The model under review builds one solid part; all positions refer to its coordinate system, in mm. A direction names the side the tool comes from. Coordinates: 2 decimals unless noted, no trailing zeros. Order: outer loops, then holes, each group sorted by start corner. A loop starts at its lowest first (then second) coordinate and runs counter-clockwise, first axis right, second up. Notation, with made-up numbers: (-36, -36) -> (18, -36) arc R23 cw to (18, -17) -> close; hole circle Ø3 at (40.5, 19.25). An arc over 180 degrees is marked (long way). Put each result on its own line as item: value.
from build123d import *

# Parameters (mm, degrees)
SKETCH1_R           = 11.875
SKETCH1_R_2         = 5
BOSS_EXTRUDE1_DEPTH = 11
CUT_EXTRUDE1_DEPTH  = 21.075638221
SKETCH4_R           = 13.875
SKETCH4_R_2         = 5
BOSS_EXTRUDE2_DEPTH = 1
LPATTERN1_COUNT     = 2
LPATTERN1_PITCH     = 12


with BuildPart() as part:
    # Sketch1 → Boss-Extrude1 (new body)
    with BuildSketch(Plane(origin=(0, 0, 0), x_dir=(0, 0, -1), z_dir=(1, 0, 0))):
        Circle(SKETCH1_R)
        Circle(SKETCH1_R_2, mode=Mode.SUBTRACT)
    extrude(amount=BOSS_EXTRUDE1_DEPTH)

    # Sketch2 → Cut-Extrude1 (cut, through all)
    with BuildSketch(Plane.ZY):
        with BuildLine():
            Line((1.26491017, 11.807439488), (0.63461115, 10.455758877))
            ThreePointArc((0.63461115, 10.455758877), (0, 10.475), (-0.63461115, 10.455758877))
            Line((-0.63461115, 10.455758877), (-1.26491017, 11.807439488))
            ThreePointArc((-1.26491017, 11.807439488), (0, 11.875), (1.26491017, 11.807439488))
        make_face()
        with BuildLine():
            Line((5.958071241, 10.272147394), (4.8324864, 9.293691419))
            ThreePointArc((4.8324864, 9.293691419), (4.260566336, 9.569388669), (3.672994133, 9.809930637))
            Line((3.672994133, 9.809930637), (3.64696536, 11.301118027))
            ThreePointArc((3.64696536, 11.301118027), (4.829997637, 10.84835231), (5.958071241, 10.272147394))
        make_face()
        with BuildLine():
            Line((9.621027667, 6.960707696), (8.194780849, 6.524660285))
            ThreePointArc((8.194780849, 6.524660285), (7.784442047, 7.009143102), (7.345505362, 7.467876269))
            Line((7.345505362, 7.467876269), (7.928247448, 8.840730592))
            ThreePointArc((7.928247448, 8.840730592), (8.824844803, 7.945925951), (9.621027667, 6.960707696))
        make_face()
        with BuildLine():
            Line((11.620421005, 2.445698402), (10.140123243, 2.627456112))
            ThreePointArc((10.140123243, 2.627456112), (9.962317008, 3.236953016), (9.747911982, 3.834558252))
            Line((9.747911982, 3.834558252), (10.838663527, 4.851700522))
            ThreePointArc((10.838663527, 4.851700522), (11.293796131, 3.669576808), (11.620421005, 2.445698402))
        make_face()
        with BuildLine():
            Line((11.610537983, -2.492194365), (10.332146207, -1.724059091))
            ThreePointArc((10.332146207, -1.724059091), (10.417616854, -1.094935653), (10.464816064, -0.461789724))
            Line((10.464816064, -0.461789724), (11.874976215, 0.023767355))
            ThreePointArc((11.874976215, 0.023767355), (11.809947507, -1.241275501), (11.610537983, -2.492194365))
        make_face()
        with BuildLine():
            Line((9.593087465, -6.999164085), (8.737647228, -5.777468816))
            ThreePointArc((8.737647228, -5.777468816), (9.071616105, -5.2375), (9.372258378, -4.678290061))
            Line((9.372258378, -4.678290061), (10.857997635, -4.808275403))
            ThreePointArc((10.857997635, -4.808275403), (10.28405167, -5.9375), (9.593087465, -6.999164085))
        make_face()
        with BuildLine():
            Line((5.916904974, -10.295914749), (5.632329664, -8.831901695))
            ThreePointArc((5.632329664, -8.831901695), (6.157050518, -8.474453016), (6.659152074, -8.085871545))
            Line((6.659152074, -8.085871545), (7.963572623, -8.808923662))
            ThreePointArc((7.963572623, -8.808923662), (6.979949871, -9.607076808), (5.916904974, -10.295914749))
        make_face()
        with BuildLine():
            Line((1.21763586, -11.812408218), (1.553131133, -10.359218536))
            ThreePointArc((1.553131133, -10.359218536), (2.177874961, -10.246096118), (2.794617881, -10.095332382))
            Line((2.794617881, -10.095332382), (3.692173556, -11.286428994))
            ThreePointArc((3.692173556, -11.286428994), (2.468951328, -11.615502759), (1.21763586, -11.812408218))
        make_face()
        with BuildLine():
            Line((-3.692173556, -11.286428994), (-2.794617881, -10.095332382))
            ThreePointArc((-2.794617881, -10.095332382), (-2.177874961, -10.246096118), (-1.553131133, -10.359218536))
            Line((-1.553131133, -10.359218536), (-1.21763586, -11.812408218))
            ThreePointArc((-1.21763586, -11.812408218), (-2.468951328, -11.615502759), (-3.692173556, -11.286428994))
        make_face()
        with BuildLine():
            Line((-7.963572623, -8.808923662), (-6.659152074, -8.085871545))
            ThreePointArc((-6.659152074, -8.085871545), (-6.157050518, -8.474453016), (-5.632329664, -8.831901695))
            Line((-5.632329664, -8.831901695), (-5.916904974, -10.295914749))
            ThreePointArc((-5.916904974, -10.295914749), (-6.979949871, -9.607076808), (-7.963572623, -8.808923662))
        make_face()
        with BuildLine():
            Line((-10.857997635, -4.808275403), (-9.372258378, -4.678290061))
            ThreePointArc((-9.372258378, -4.678290061), (-9.071616105, -5.2375), (-8.737647228, -5.777468816))
            Line((-8.737647228, -5.777468816), (-9.593087465, -6.999164085))
            ThreePointArc((-9.593087465, -6.999164085), (-10.28405167, -5.9375), (-10.857997635, -4.808275403))
        make_face()
        with BuildLine():
            Line((-11.874976215, 0.023767355), (-10.464816064, -0.461789724))
            ThreePointArc((-10.464816064, -0.461789724), (-10.417616854, -1.094935653), (-10.332146207, -1.724059091))
            Line((-10.332146207, -1.724059091), (-11.610537983, -2.492194365))
            ThreePointArc((-11.610537983, -2.492194365), (-11.809947507, -1.241275501), (-11.874976215, 0.023767355))
        make_face()
        with BuildLine():
            Line((-10.838663527, 4.851700522), (-9.747911982, 3.834558252))
            ThreePointArc((-9.747911982, 3.834558252), (-9.962317008, 3.236953016), (-10.140123243, 2.627456112))
            Line((-10.140123243, 2.627456112), (-11.620421005, 2.445698402))
            ThreePointArc((-11.620421005, 2.445698402), (-11.293796131, 3.669576808), (-10.838663527, 4.851700522))
        make_face()
        with BuildLine():
            Line((-7.928247448, 8.840730592), (-7.345505362, 7.467876269))
            ThreePointArc((-7.345505362, 7.467876269), (-7.784442047, 7.009143102), (-8.194780849, 6.524660285))
            Line((-8.194780849, 6.524660285), (-9.621027667, 6.960707696))
            ThreePointArc((-9.621027667, 6.960707696), (-8.824844803, 7.945925951), (-7.928247448, 8.840730592))
        make_face()
        with BuildLine():
            Line((-3.64696536, 11.301118027), (-3.672994133, 9.809930637))
            ThreePointArc((-3.672994133, 9.809930637), (-4.260566336, 9.569388669), (-4.8324864, 9.293691419))
            Line((-4.8324864, 9.293691419), (-5.958071241, 10.272147394))
            ThreePointArc((-5.958071241, 10.272147394), (-4.829997637, 10.84835231), (-3.64696536, 11.301118027))
        make_face()
    extrude(amount=-CUT_EXTRUDE1_DEPTH, mode=Mode.SUBTRACT)

    # Sketch4 → Boss-Extrude2 (add)
    with BuildSketch(Plane(origin=(11, 0, 0), x_dir=(0, 0, -1), z_dir=(1, 0, 0))):
        Circle(SKETCH4_R)
        Circle(SKETCH4_R_2, mode=Mode.SUBTRACT)
    boss_extrude2 = extrude(amount=BOSS_EXTRUDE2_DEPTH)

    # LPattern1: Boss-Extrude2 ×2
    with Locations(*[(-i * LPATTERN1_PITCH, 0, 0) for i in range(1, LPATTERN1_COUNT)]):
        add(boss_extrude2)


solid = part.part
Item 1: For faces 1 (the flat face through (5.42, 8.16, -7.64)), 2 (the flat face through (5.42, 4.34, 10.29)), 3 (the cylindrical face through (5.42, -3.65, 11.3)), 4 (the flat face through (5.423, 11.122, -0.945)), list the 3-axis set-ups (+Z, -Z, +X, -X, +Y, -Y) from which the entire face can be reached by the end or side of a thin tool; tool diameter is ignored.
Answers below:
face 1: -Z
face 2: +Z
face 3: +Z, -Y
face 4: +Y
Item 2: Consider section D-D on y = 6. Write out the cut boundary in (x, z).
Answers below:
outline: (-1, -12.51) -> (0, -12.51) -> (0, -10.25) -> (11, -10.25) -> (11, -12.51) -> (12, -12.51) -> (12, 12.51) -> (11, 12.51) -> (11, 10.25) -> (0, 10.25) -> (0, 12.51) -> (-1, 12.51) -> close
Item 3: Consider section C-C on y = -7.75. Write out the cut boundary in (x, z), and give its area (3 significant figures).
Answers below:
outline: (-1, -11.51) -> (0, -11.51) -> (0, -9) -> (11, -9) -> (11, -11.51) -> (12, -11.51) -> (12, 11.51) -> (11, 11.51) -> (11, 9) -> (0, 9) -> (0, 11.51) -> (-1, 11.51) -> close
area: 244 mm^2
Item 4: Mouldability with a two-part tool opening along X and no side actions: class faces 5 (the flat face through (5.42, 8.14, 7.63)), 6 (the cylindrical face through (5.41, -4.88, 1.08)) as +X half, -X half, draft (parallel to the pull), parting line (faces both ways), or undercut.
Answers below:
face 5: undercut
face 6: draft
Item 5: Consider section A-A on z = 0. Write out the cut boundary in (x, y) (3 decimals), and give its area (3 significant figures).
Answers below:
outline: (-1, -13.875) -> (0, -13.875) -> (0, -11.875) -> (11, -11.875) -> (11, -13.875) -> (12, -13.875) -> (12, -5) -> (-1, -5) -> close; (-1, 5) -> (12, 5) -> (12, 13.875) -> (11, 13.875) -> (11, 10.475) -> (0, 10.475) -> (0, 13.875) -> (-1, 13.875) -> close
area: 171 mm^2
Item 6: For line 1 (X direction, y = -2.25, z = 11.5); line 2 (Y direction, x = 4.5, z = 0) (3 decimals); line 3 (Y direction, x = 3.75, z = -10.5), list the stretches that pass through material, from the lowest coordinate up. Write a range as from..to.
Answers below:
line 1: -1..0, 11..12
line 2: -11.875..-5, 5..10.475
line 3: -4.78..-1.82, -0.45..2.58, 4.54..5.55
Item 7: Consider section B-B on y = 1.75. Write out the cut boundary in (x, z).
Answers below:
outline: (-1, -13.76) -> (0, -13.76) -> (0, -11.75) -> (11, -11.75) -> (11, -13.76) -> (12, -13.76) -> (12, -4.68) -> (-1, -4.68) -> close; (-1, 4.68) -> (12, 4.68) -> (12, 13.76) -> (11, 13.76) -> (11, 11.75) -> (0, 11.75) -> (0, 13.76) -> (-1, 13.76) -> close
Item 8: For pin 1 Ø2 at (x, y) = (3.5, 4.5) entering from -Z; pin 2 Ø3 at (x, y) = (0.5, 2) entering from -Z; pin 3 Ø5 at (x, y) = (5.5, -1.5) entering from +Z (3 decimals), all flat-tipped, find the tip position at first contact; note any pin that passes through.
Answers below:
pin 1: z = -10.84
pin 2: z = -13.86
pin 3: z = 11.875
